Autodesk Inventor part; units mm, degrees
ref_plane "Work Plane1" through (0, 0, 0) normal (0, 0, 1) x (1, 0, 0)
ref_plane "YZ Plane" through (0, 0, 0) normal (1, 0, 0) x (0, 1, 0)
ref_plane "XZ Plane" through (0, 0, 0) normal (0, 1, 0) x (-1, 0, 0)
ref_plane "Work Plane1" through (0, 0, 0) normal (0, 0, 1) x (1, 0, 0)
sketch "Sketch1" plane through (0, 0, 0) normal (0, 0, 1) x (1, 0, 0)
  line L0 (272, -4) -> (-8, -4) construction
  line L1 (230, 0) -> (230, -3.492) construction
  line L2 (272, 102.8084) -> (-8, 102.8084) construction
  line L3 (62, 0) -> (62, -4) construction
  line L4 (78, 0) -> (78, -3.492) construction
  circle A0 centre (220, 0) radius 2 construction
  circle A1 centre (164, 0) radius 2 construction
  circle A2 centre (148, 0) radius 2 construction
  circle A3 centre (140, 0) radius 2 construction
  circle A4 centre (132, 0) radius 2 construction
  circle A5 centre (124, 0) radius 2 construction
  circle A6 centre (116, 0) radius 2 construction
  circle A7 centre (116, 98.8084) radius 2 construction
  circle A8 centre (124, 98.8084) radius 2 construction
  circle A9 centre (132, 98.8084) radius 2 construction
  circle A10 centre (140, 98.8084) radius 2 construction
  circle A11 centre (148, 98.8084) radius 2 construction
  circle A12 centre (156, 98.8084) radius 2 construction
  circle A13 centre (164, 98.8084) radius 2 construction
  circle A14 centre (172, 98.8084) radius 2 construction
  circle A15 centre (180, 98.8084) radius 2 construction
  circle A16 centre (188, 98.8084) radius 2 construction
  circle A17 centre (196, 98.8084) radius 2 construction
  circle A18 centre (204, 98.8084) radius 2 construction
  circle A19 centre (212, 98.8084) radius 2 construction
  circle A20 centre (220, 98.8084) radius 2 construction
  circle A21 centre (212, 0) radius 2 construction
  circle A22 centre (204, 0) radius 2 construction
  circle A23 centre (196, 0) radius 2 construction
  circle A24 centre (188, 0) radius 2 construction
  circle A25 centre (180, 0) radius 2 construction
  circle A26 centre (172, 0) radius 2 construction
  circle A27 centre (156, 0) radius 2 construction
  circle A28 centre (220, 0) radius 2.2479
  circle A29 centre (211.999, 0) radius 2.2479
  circle A30 centre (203.998, 0) radius 2.2479
  circle A31 centre (195.997, 0) radius 2.2479
  circle A32 centre (187.996, 0) radius 2.2479
  circle A33 centre (179.995, 0) radius 2.2479
  circle A34 centre (171.994, 0) radius 2.2479
  circle A35 centre (163.993, 0) radius 2.2479
  circle A36 centre (155.992, 0) radius 2.2479
  circle A37 centre (147.991, 0) radius 2.2479
  circle A38 centre (139.99, 0) radius 2.2479
  circle A39 centre (131.989, 0) radius 2.2479
  circle A40 centre (123.988, 0) radius 2.2479
  circle A41 centre (115.987, 0) radius 2.2479
  circle A42 centre (220, 98.8084) radius 2.2479
  circle A43 centre (211.999, 98.8084) radius 2.2479
  circle A44 centre (203.998, 98.8084) radius 2.2479
  circle A45 centre (195.997, 98.8084) radius 2.2479
  circle A46 centre (187.996, 98.8084) radius 2.2479
  circle A47 centre (179.995, 98.8084) radius 2.2479
  circle A48 centre (171.994, 98.8084) radius 2.2479
  circle A49 centre (163.993, 98.8084) radius 2.2479
  circle A50 centre (155.992, 98.8084) radius 2.2479
  circle A51 centre (147.991, 98.8084) radius 2.2479
  circle A52 centre (139.99, 98.8084) radius 2.2479
  circle A53 centre (131.989, 98.8084) radius 2.2479
  circle A54 centre (123.988, 98.8084) radius 2.2479
  circle A55 centre (115.987, 98.8084) radius 2.2479
  line L5 (106.175, 30.29) -> (106.175, -3.492) construction
  line L6 (227.46, -3.492) -> (227.46, 102.3004) construction
  line L7 (106.175, 102.3004) -> (106.175, 69.6341) construction
  line L8 (205, 69.6341) -> (205, 30.29) construction
  line L9 (205, 69.6341) -> (205, 30.29) construction
  line L10 (106.175, 102.3004) -> (227.46, 102.3004)
  line L11 (227.46, 102.3004) -> (227.46, -3.492)
  line L12 (227.46, -3.492) -> (106.175, -3.492)
  line L13 (106.175, -3.492) -> (106.175, 30.29)
  line L14 (106.175, 30.29) -> (205, 30.29)
  line L15 (205, 30.29) -> (205, 69.6341)
  line L16 (205, 69.6341) -> (106.175, 69.6341)
  line L17 (106.175, 69.6341) -> (106.175, 102.3004)
  point P0 (0, 0)
  point P1 (-8, -4)
  dimension "d0" = 4.4958
  dimension "d3" = 8.001
  dimension "d8" = 4.4958
  dimension "d11" = 8.001
extrude "Extrusion2" add sketch "Sketch1" along normal blind 2.54
properties part number "Flat Roof panel"
Model file for the job. Use its own axes, mm. A direction names the side the tool comes from. Coordinates: 2 decimals unless noted, no trailing zeros. Write each loop counter-clockwise with the first axis right and the second up, starting at its lowest first coordinate (ties: lowest second). Pieces come first, ordered by that corner, then holes. Notation, with made-up numbers: (62.5, 18.25) - (121.5, 18.25) arc R35 cw to (121.5, 50.25) - close; hole circle Ø7 at (11.5, -32). An arc over 180 degrees is marked (long way). One line per item, written item: value. Start each with the question number.
1. Slice it at A-A (x = 139.99). Write the cut outline in (y, z).
2. Mould opens along Y. For faces 3 (the cylindrical face through (209.753, -0.099, 1.252)), 4 (the cylindrical face through (118.13, 98.13, 1.25)), 5 (the flat face through (227.46, 50, 1)), 6 (the flat face through (166, 102.3, 1)) say: released by +Y, released by -Y, zero draft, split by the parting line, or undercut.
3. Probe line 1 (Y direction, x = 220, z = 0.85); line 2 (Y direction, x = 140, z = 0.85); line 3 (Y direction, x = 167, z = 1.75). List the from-to ranges inside material, lowest first. Write a range as from..to.
4. Slice it at D-D (y = 48). Write the cut outline in (x, z), plus the area to 3 significant figures.
5. Slice it at C-C (y = 0). Count the separate pieces of the cut face and the enclosed holes in it, plus the area to 3 significant figures.
6. Tool access for faces 1 (the cylindrical face through (185.75, 98.71, 1.25)), 2 (the flat face through (156, 69.634, 1)): list every direction of +Z, -Z, +X, -X, +Y, -Y with a clear straight run to the whole face (end or side of a thin tool).
7. Flat gauge pin, fed straight in: pin 1 (1 mm diameter, centred on y = 35, z = 1.5, fed in from -X). Where does the tip first touch, or does it go through?
8. Slice it at B-B (x = 220). Write the cut outline in (y, z).
Answers below:
1. outline: (-3.49, 0) - (-2.25, 0) - (-2.25, 2.54) - (-3.49, 2.54) - close; (2.25, 0) - (30.29, 0) - (30.29, 2.54) - (2.25, 2.54) - close; (69.63, 0) - (96.56, 0) - (96.56, 2.54) - (69.63, 2.54) - close; (101.06, 0) - (102.3, 0) - (102.3, 2.54) - (101.06, 2.54) - close
2. face 3: undercut
2. face 4: undercut
2. face 5: zero draft
2. face 6: released by +Y
3. line 1: y = -3.49..-2.25, 2.25..96.56, 101.06..102.3
3. line 2: y = -3.49..-2.25, 2.25..30.29, 69.63..96.56, 101.06..102.3
3. line 3: y = -3.49..30.29, 69.63..102.3
4. outline: (205, 0) - (227.46, 0) - (227.46, 2.54) - (205, 2.54) - close
4. area: 57.0 mm^2
5. separate pieces: 15
5. enclosed holes: 0
5. area: 148 mm^2
6. face 1: +Z, -Z
6. face 2: +Z, -Z, -X
7. pin 1: stops at x = 205
8. outline: (-3.49, 0) - (-2.25, 0) - (-2.25, 2.54) - (-3.49, 2.54) - close; (2.25, 0) - (96.56, 0) - (96.56, 2.54) - (2.25, 2.54) - close; (101.06, 0) - (102.3, 0) - (102.3, 2.54) - (101.06, 2.54) - close
